Input: dimensioned drawing with shaded views. Units: mm. Origin: part minimum x, y, z. Coordinates: 2 decimals unless noted, no trailing zeros. Write each loop counter-clockwise with the first axis right and the second up, starting at its lowest first coordinate (ties: lowest second). Pieces come first, ordered by that corner, then holes. Notation, with made-up numbers: (53.25, 67.5) - (66.25, 67.5) arc R18 ccw to (66.25, 75.5) - close; hole circle Ø5 at (71.5, 79). An arc over 180 degrees is marked (long way). One line per question, with ' | ' between items.
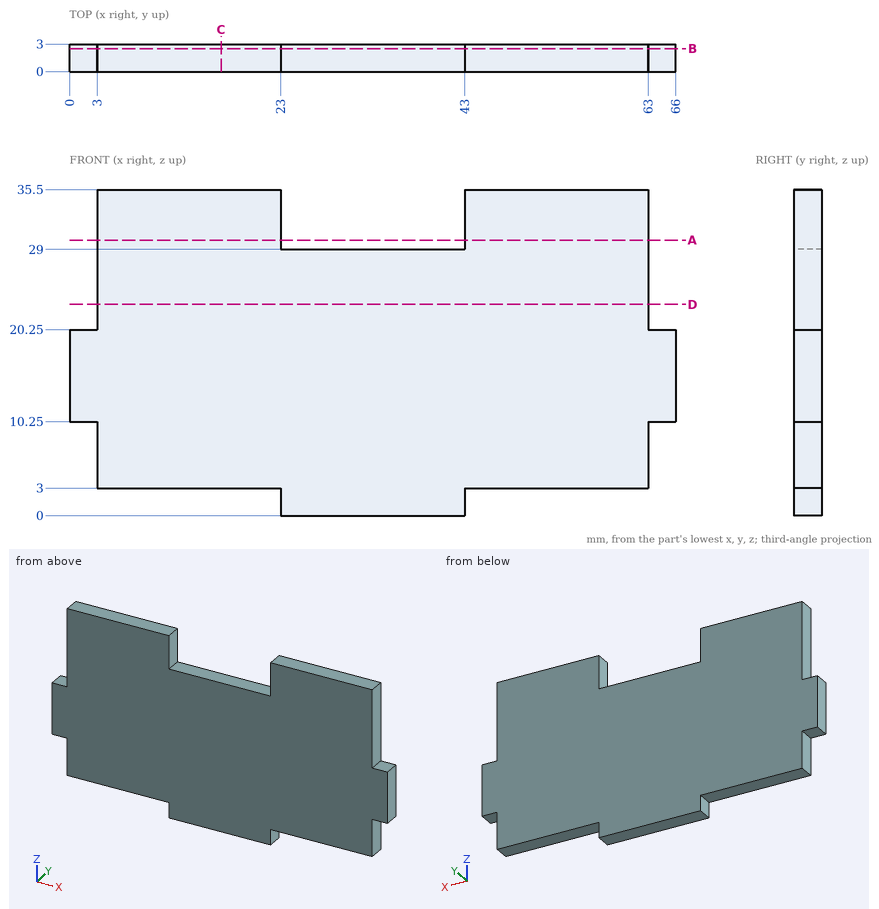
Item 1: Cut plane D-D on z = 23. Return loops of the section in (x, y), and give its area (3 significant figures).
Check sheet entries:
outline: (3, 0) - (63, 0) - (63, 3) - (3, 3) - close | area: 180 mm²
Item 2: Cut plane A-A on z = 30. Return loops of the section in (x, y), and give its area (3 significant figures).
Check sheet entries:
outline: (3, 0) - (23, 0) - (23, 3) - (3, 3) - close; (43, 0) - (63, 0) - (63, 3) - (43, 3) - close | area: 120 mm²
Item 3: Pin query (flat end, axial travel): pin 1 Ø0.9 at (x, y) = (65, 1) entering from -Z; pin 2 Ø1.5 at (y, z) = (1, 8) entering from -X; pin 3 Ø0.9 at (x, y) = (51.5, 2) entering from -Z. Return the tip coordinate at first contact, or that it passes through.
Check sheet entries:
pin 1: z = 10.25 | pin 2: x = 3 | pin 3: z = 3
Item 4: Cut plane C-C on x = 16.5. Return loops of the section in (y, z), and give its area (3 significant figures).
Check sheet entries:
outline: (0, 3) - (3, 3) - (3, 35.5) - (0, 35.5) - close | area: 97.5 mm²
Item 5: Cut plane B-B on y = 2.5. Return loops of the section in (x, z).
Check sheet entries:
outline: (0, 10.25) - (3, 10.25) - (3, 3) - (23, 3) - (23, 0) - (43, 0) - (43, 3) - (63, 3) - (63, 10.25) - (66, 10.25) - (66, 20.25) - (63, 20.25) - (63, 35.5) - (43, 35.5) - (43, 29) - (23, 29) - (23, 35.5) - (3, 35.5) - (3, 20.25) - (0, 20.25) - close
Item 6: Ray query, line 1 along X through (y, z) = (0.45, 30); line 2 along Z through (x, y) = (26, 2.45); line 3 along X through (y, z) = (2.2, 22). Return the intervals inside material, ascending. Write a range as [from, to].
Check sheet entries:
line 1: [3, 23], [43, 63] | line 2: [0, 29] | line 3: [3, 63]
